Could you check a few things on this model? Use its own coordinates, in mm. Coordinates: 2 decimals unless noted, no trailing zeros. Loops run counter-clockwise (first coordinate to the right, second up) from the corner with the lowest first, then second, coordinate; pieces in that order, holes last. Notation, with made-up numbers: (84.25, 45.5) -> (131.25, 45.5) arc R27 ccw to (131.25, 82.5) -> close; hole circle Ø11 at (12, 56.25). An arc over 180 degrees is marked (long way). One line per question, with ' | ' between items. Start each with the question number.
(1) Suppose I cut it at D-D (x = -12). Please give me the cut outline in (y, z) (3 decimals).
(2) Suppose I cut it at C-C (z = 64). Please give me the cut outline in (x, y) (3 decimals).
(3) Suppose I cut it at B-B (y = 2.3). Please give me the cut outline in (x, z).
(4) If we mould it in two halves opening along X, with no side actions, what happens to faces 1 (the face through (41.07, 1.57, 72.49)), 2 (the face through (-42.239, 1.565, 71.814)), 3 (the face through (0.11, 1.565, 61.636))? For each: pulls with the +X half, pulls with the -X half, needs draft (parallel to the pull), parting line crosses it, or undercut.
(5) Suppose I cut it at A-A (z = 0). Please give me the cut outline in (x, y) (3 decimals), plus the area to 3 significant figures.
(6) If I drill on line 1 along Z through (x, y) = (55, 0.45); line 2 along Z through (x, y) = (55.5, 1); line 3 along X through (y, z) = (1.35, 1.5), over which ranges is the centre line in solid material (lowest first)?
(7) I'm going to push flat-ended pins straight in: pin 1 Ø5 at (x, z) = (0, 0) entering from +Y; pin 2 Ø1 at (y, z) = (1, 76.5) entering from -X; pin 3 Ø1 at (x, y) = (59.5, 1) entering from +Z; pin 4 Ø1 at (x, y) = (-23.5, 2) entering from +Z. Where does each tip first touch, or does it pass through?
```python
from build123d import *

# Parameters (mm, degrees)
SKETCH2_R           = 3.96875
SKETCH2_R_2         = 2.5
BOSS_EXTRUDE1_DEPTH = 3.175


with BuildPart() as part:
    # Sketch2 → Boss-Extrude1 (new body)
    with BuildSketch(Plane(origin=(0, 0, 0), x_dir=(1, 0, 0), z_dir=(0, 1, 0))):
        Polygon((83.312, -48.100205627), (83.312, 48.100205627), (0, 96.200411253), (-83.312, 48.100205627), (-83.312, -48.100205627), (0, -96.200411253), align=None)
        with Locations(Location((0, 0, 0), (0, 0, 270))):
            Circle(SKETCH2_R, mode=Mode.SUBTRACT)
        with Locations(Location((-55.541333303, 32.066803734, 0), (0, 0, 270))):
            Circle(SKETCH2_R_2, mode=Mode.SUBTRACT)
        with Locations(Location((0, 64.133607467, 0), (0, 0, 270))):
            Circle(SKETCH2_R_2, mode=Mode.SUBTRACT)
        with Locations(Location((55.541333303, 32.066803734, 0), (0, 0, 270))):
            Circle(SKETCH2_R_2, mode=Mode.SUBTRACT)
        with Locations(Location((55.541333303, -32.066803734, 0), (0, 0, 270))):
            Circle(SKETCH2_R_2, mode=Mode.SUBTRACT)
        with Locations(Location((0, -64.133607467, 0), (0, 0, 270))):
            Circle(SKETCH2_R_2, mode=Mode.SUBTRACT)
        with Locations(Location((-55.541333303, -32.066803734, 0), (0, 0, 270))):
            Circle(SKETCH2_R_2, mode=Mode.SUBTRACT)
    extrude(amount=BOSS_EXTRUDE1_DEPTH)


solid = part.part
```
Checks:
1) outline: (0, -89.272) -> (3.175, -89.272) -> (3.175, 89.272) -> (0, 89.272) -> close
2) outline: (-55.773, 0) -> (-2.496, 0) -> (-2.496, 3.175) -> (-55.773, 3.175) -> close; (2.496, 0) -> (55.773, 0) -> (55.773, 3.175) -> (2.496, 3.175) -> close
3) outline: (-83.31, -48.1) -> (0, -96.2) -> (83.31, -48.1) -> (83.31, 48.1) -> (0, 96.2) -> (-83.31, 48.1) -> close; hole circle Ø5 at (-55.54, -32.07); hole circle Ø5 at (-55.54, 32.07); hole circle Ø7.94 at (0, 0); hole circle Ø5 at (0, -64.13); hole circle Ø5 at (0, 64.13); hole circle Ø5 at (55.54, -32.07); hole circle Ø5 at (55.54, 32.07)
4) face 1: pulls with the +X half | face 2: pulls with the -X half | face 3: undercut
5) outline: (-83.312, 0) -> (-3.969, 0) -> (-3.969, 3.175) -> (-83.312, 3.175) -> close; (3.969, 0) -> (83.312, 0) -> (83.312, 3.175) -> (3.969, 3.175) -> close | area: 504 mm^2
6) line 1: z = -64.45 to -34.51, -29.63 to 29.63, 34.51 to 64.45 | line 2: z = -64.16 to -34.57, -29.57 to 29.57, 34.57 to 64.16 | line 3: x = -83.31 to -3.67, 3.67 to 83.31
7) pin 1: passes through | pin 2: stops at x = -34.99 | pin 3: stops at z = 62.14 | pin 4: stops at z = 82.92
